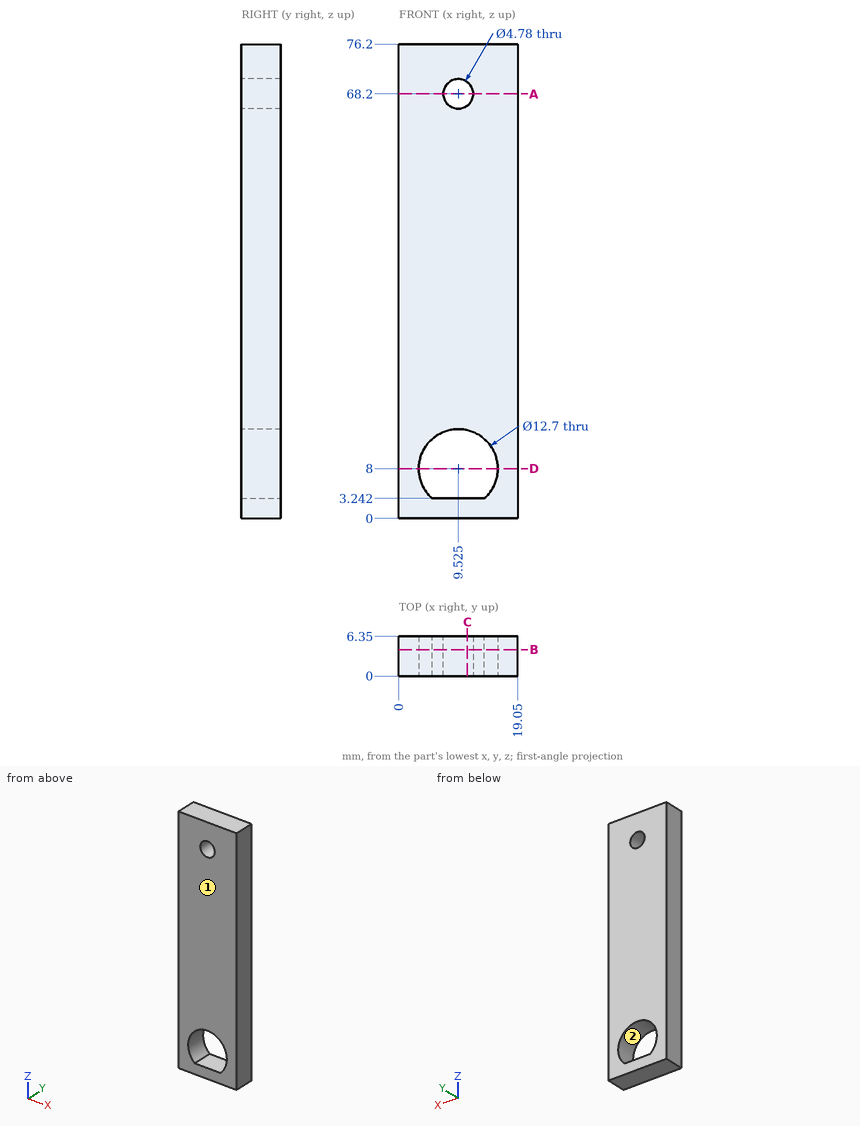
Part print with two shaded views. Sizes in mm from the minimum x, y, z corner. Give positions to 0.01 mm unless a question says otherwise; leave off trailing zeros. Order: outer loops, then holes, each group sorted by start corner. A loop starts at its lowest first (then second) coordinate and runs counter-clockwise, first axis right, second up. Notation, with made-up numbers: M -1,-17.75 L 46,-17.75 A12 cw 46,-5.75 Z; hole C -26,-4.75 d8. An arc over 180 degrees is marked long. Write item = value, one per line.
Q1. Cut at D-D, the plane z = 8. List the corners of the cut face in (x, y) (3 decimals), then the cut area to 3 significant figures.
Derived:
outline = M 0,0 L 3.175,0 L 3.175,6.35 L 0,6.35 Z; M 15.875,0 L 19.05,0 L 19.05,6.35 L 15.875,6.35 Z
area = 40.3 mm2
Q2. Drill centre lines: line 1 (X direction, y = 3.5, z = 68.2) (3 decimals); line 2 (X direction, y = 4.75, z = 8) (3 decimals); line 3 (Z direction, x = 11.5, y = 2) (1 decimal). Where is each one in solid material? Low to high. Write a range as [from, to].
Derived:
line_1 = [0, 7.135], [11.915, 19.05]
line_2 = [0, 3.175], [15.875, 19.05]
line_3 = [0, 3.2], [14, 66.9], [69.5, 76.2]
Q3. Cut at B-B, the plane y = 4.25. Count the separate pieces of the cut face and the enclosed holes in it, then the cut area to 3 significant figures.
Derived:
separate_pieces = 1
enclosed_holes = 2
area = 1,320 mm2
Q4. Cut at C-C, the plane x = 11. List the corners of the cut face in (y, z).
Derived:
outline = M 0,0 L 6.35,0 L 6.35,3.24 L 0,3.24 Z; M 0,14.18 L 6.35,14.18 L 6.35,66.32 L 0,66.32 Z; M 0,70.08 L 6.35,70.08 L 6.35,76.2 L 0,76.2 Z
Q5. Cut at A-A, the plane z = 68.2. List the corners of the cut face in (x, y) (3 decimals), then the cut area to 3 significant figures.
Derived:
outline = M 0,0 L 7.135,0 L 7.135,6.35 L 0,6.35 Z; M 11.915,0 L 19.05,0 L 19.05,6.35 L 11.915,6.35 Z
area = 90.6 mm2
Q6. Flat gauge pins, fed straight in: pin 1 (4 mm diameter, centred on x = 15.5, z = 60, fed in from -Y); pin 2 (7.5 mm diameter, centred on x = 9.525, z = 8, fed in from +Y). Where does each tip first touch, or does it go through?
Derived:
pin_1 = 0
pin_2 = through
Q7. Two-plate mould, pull along X, no slides. Class the marked faces 1 and 2: pulls with the +X half, pulls with the -X half, needs draft (parallel to the pull), parting line crosses it, or undercut.
Derived:
face_1 = needs draft
face_2 = undercut
